Geometry: final body of the model. Coordinates: model frame, mm. Coordinates: 2 decimals unless noted, no trailing zeros. Loops run counter-clockwise (first coordinate to the right, second up) from the corner with the lowest first, then second, coordinate; pieces in that order, holes last. Notation, with made-up numbers: (23, 16.25) -> (28, 16.25) arc R27 cw to (28, 45.25) -> close; hole circle Ø8 at (75.5, -24). An arc over 180 degrees is marked (long way). One line per item, written item: value. Start each with the question number.
Item 1: Section query D-D on y = -94.5. Return loops of the section in (x, z), then the cut area to 3 significant figures.
Item 2: Ray query, probe 1 along Y at (x, z) = (8, 1.15); probe 2 along X at (y, z) = (9.5, 3.35) (3 decimals); probe 3 along Y at (x, z) = (4.5, 0.7). Return the intervals inside material, ascending. Write a range as from..to.
Item 3: Section query A-A on y = 0. Return loops of the section in (x, z) (3 decimals).
Item 4: Contact query for a flat-ended pin moving along its axis: pin 1 Ø2 at (y, z) = (-159.5, 1.5) entering from +X. Output: stop coordinate, or through.
Item 5: Section query C-C on z = 3.2. Return loops of the section in (x, y) (3 decimals).
Item 6: Section query B-B on x = 0. Return loops of the section in (y, z).
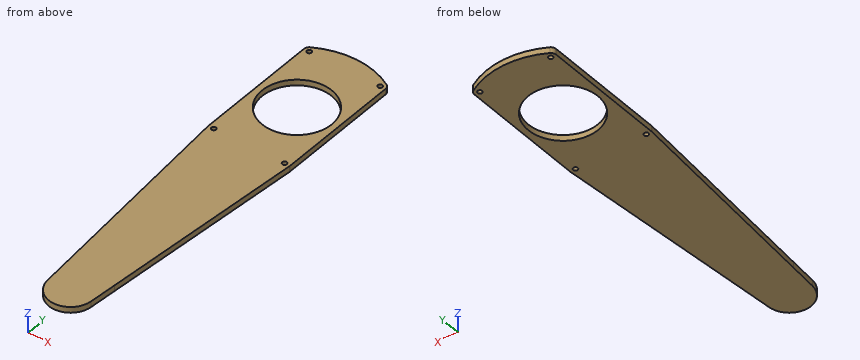
from build123d import *

# Parameters (mm, degrees)
SKETCH1_R           = 1.55
SKETCH1_R_2         = 24
BOSS_EXTRUDE1_DEPTH = 4
SKETCH1_4_R         = 15
BOSS_EXTRUDE2_DEPTH = 4


with BuildPart() as part:
    # Sketch1 → Boss-Extrude1 (new body)
    with BuildSketch(Plane.XY):
        with BuildLine():
            ThreePointArc((-26.25, 45.466333699), (-27.622595264, 44.093738434), (-28.125, 42.218738434))
            Line((-28.125, 42.218738434), (-28.125, -42.218738434))
            ThreePointArc((-28.125, -42.218738434), (-28.12179062, -42.373851469), (-28.112167971, -42.528699002))
            ThreePointArc((-28.112167971, -42.528699002), (-27.542259342, -44.226465573), (-26.25, -45.466333699))
            ThreePointArc((-26.25, -45.466333699), (0, -52.5), (26.25, -45.466333699))
            ThreePointArc((26.25, -45.466333699), (27.542259342, -44.226465573), (28.112167971, -42.528699002))
            ThreePointArc((28.112167971, -42.528699002), (28.12179062, -42.373851469), (28.125, -42.218738434))
            Line((28.125, -42.218738434), (28.125, 42.218738434))
            ThreePointArc((28.125, 42.218738434), (27.622595264, 44.093738434), (26.25, 45.466333699))
            ThreePointArc((26.25, 45.466333699), (0, 52.5), (-26.25, 45.466333699))
        make_face()
        with Locations((-24.375, -42.218738434)):
            Circle(SKETCH1_R, mode=Mode.SUBTRACT)
        with Locations((-24.375, 42.218738434)):
            Circle(SKETCH1_R, mode=Mode.SUBTRACT)
        Circle(SKETCH1_R_2, mode=Mode.SUBTRACT)
        with Locations((24.375, -42.218738434)):
            Circle(SKETCH1_R, mode=Mode.SUBTRACT)
        with Locations((24.375, 42.218738434)):
            Circle(SKETCH1_R, mode=Mode.SUBTRACT)
    extrude(amount=BOSS_EXTRUDE1_DEPTH)

    # Sketch1_4 → Boss-Extrude2 (add)
    with BuildSketch(Plane.XY):
        with BuildLine():
            ThreePointArc((-26.25, -45.466333699), (-27.542259342, -44.226465573), (-28.112167971, -42.528699002))
            Line((-28.112167971, -42.528699002), (-16.497234382, -182.568957067))
            ThreePointArc((-16.497234382, -182.568957067), (0, -176), (16.497234382, -182.568957067))
            Line((16.497234382, -182.568957067), (28.112167971, -42.528699002))
            ThreePointArc((28.112167971, -42.528699002), (27.542259342, -44.226465573), (26.25, -45.466333699))
            ThreePointArc((26.25, -45.466333699), (0, -52.5), (-26.25, -45.466333699))
        make_face()
        with BuildLine():
            ThreePointArc((16.497234382, -182.568957067), (0, -176), (-16.497234382, -182.568957067))
            Line((-16.497234382, -182.568957067), (-14.948671886, -201.239842268))
            ThreePointArc((-14.948671886, -201.239842268), (-0.620452139, -185.012837522), (15, -200))
            ThreePointArc((15, -200), (14.987162478, -200.620452139), (14.948671886, -201.239842268))
            Line((14.948671886, -201.239842268), (16.497234382, -182.568957067))
        make_face()
        with Locations((0, -200)):
            Circle(SKETCH1_4_R)
    extrude(amount=BOSS_EXTRUDE2_DEPTH)


solid = part.part
Reply:
1. outline: (-23.8, 0) -> (23.8, 0) -> (23.8, 4) -> (-23.8, 4) -> close
1. area: 190 mm²
2. probe 1: y = -212.69..-22.63, 22.63..51.89
2. probe 2: x = -28.125..-22.04, 22.04..28.125
2. probe 3: y = -214.31..-23.57, 23.57..52.31
3. outline: (-28.125, 0) -> (-24, 0) -> (-24, 4) -> (-28.125, 4) -> close; (24, 0) -> (28.125, 0) -> (28.125, 4) -> (24, 4) -> close
4. pin 1: stops at x = 18.49
5. outline: (-28.125, -42.219) arc R3.75 ccw to (-28.112, -42.529) -> (-14.949, -201.24) arc R15 ccw to (14.949, -201.24) -> (28.112, -42.529) arc R3.75 ccw to (28.125, -42.219) -> (28.125, 42.219) arc R3.75 ccw to (26.25, 45.466) arc R52.5 ccw to (-26.25, 45.466) arc R3.75 ccw to (-28.125, 42.219) -> close; hole circle Ø3.1 at (-24.375, -42.219); hole circle Ø3.1 at (-24.375, 42.219); hole circle Ø48 at (0, 0); hole circle Ø3.1 at (24.375, -42.219); hole circle Ø3.1 at (24.375, 42.219)
6. outline: (-215, 0) -> (-24, 0) -> (-24, 4) -> (-215, 4) -> close; (24, 0) -> (52.5, 0) -> (52.5, 4) -> (24, 4) -> close
